Autodesk Inventor part; units mm, degrees
ref_plane "YZ Plane" through (0, 0, 0) normal (1, 0, 0) x (0, 1, 0)
ref_plane "XZ Plane" through (0, 0, 0) normal (0, 1, 0) x (-1, 0, 0)
ref_plane "XY Plane" through (0, 0, 0) normal (0, 0, 1) x (1, 0, 0)
sketch "Эскиз1" plane through (0, 0, 0) normal (0, 0, 1) x (1, 0, 0)
  line L0 (0, 0) -> (45, 0)
  line L1 (45, 0) -> (45, 20)
  line L2 (45, 20) -> (0, 20)
  line L3 (0, 20) -> (0, 0)
  dimension "d0" = 45
  dimension "d1" = 20
extrude "Выдавливание1" add sketch "Эскиз1" along normal blind 1.2
sketch "Эскиз2" plane through (0, 0, 1.2) normal (0, 0, 1) x (1, 0, 0)
  line L0 (0, 20) -> (0, 0)
  line L1 (0, 10) -> (1.5, 10)
  line L2 (1.5, 10) -> (9.5, 10)
  circle A0 centre (9.5, 10) radius 8
  line L3 (45, 20) -> (0, 20)
  line L4 (22.5, 20) -> (22.5, 0)
  line L5 (0, 0) -> (45, 0)
  circle A1 centre (35.5, 10) radius 8
  dimension "d5" = 16
  dimension "d4" = 1.5
extrude "Выдавливание2" add sketch "Эскиз2" along normal blind 13.8 contours A0 | A1
sketch "Эскиз3" plane through (0, 0, 1.2) normal (0, 0, 1) x (1, 0, 0)
  line L0 (45, 20) -> (0, 20)
  line L1 (22.5, 20) -> (22.5, 19.5)
  line L2 (27.5, 17.75) -> (17.5, 17.75) construction
  line L3 (25.75, 19.5) -> (19.25, 19.5)
  line L4 (19.25, 16) -> (25.75, 16)
  arc A0 (25.75, 16) -> (25.75, 19.5) centre (25.75, 17.75) ccw
  arc A1 (19.25, 19.5) -> (19.25, 16) centre (19.25, 17.75) ccw
  point P0 (0, 0)
  point P1 (22.5, 17.75)
  dimension "d8" = 0.5
  dimension "d9" = 10
  dimension "d10" = 3.5
extrude "Выдавливание3" add sketch "Эскиз3" along normal blind 3.3
sketch "Эскиз8" plane through (0, 0, 0) normal (0, 0, -1) x (-1, 0, 0)
  line L0 (-45, 0) -> (-45, 20)
  line L1 (-45, 20) -> (-44, 20)
  line L2 (-45, 20) -> (0, 20)
  line L3 (-44, 20) -> (-44, 19)
  circle A0 centre (-44, 19) radius 0.5
  line L4 (-45, 10) -> (0, 10)
  line L5 (0, 20) -> (0, 0)
  line L6 (-22.5, 20) -> (-22.5, 0)
  line L7 (0, 0) -> (-45, 0)
  circle A1 centre (-44, 1) radius 0.5
  circle A2 centre (-1, 19) radius 0.5
  circle A3 centre (-1, 1) radius 0.5
  dimension "d41" = 1
  dimension "d42" = 1
  dimension "d43" = 1
extrude "Выдавливание8" cut sketch "Эскиз8" against normal through all contours A0 | A1 | A2 | A3
sketch "Эскиз4" plane through (0, 0, 0) normal (0, 0, -1) x (-1, 0, 0)
  line L0 (-27.5, 2.5) -> (-17.5, 2.5)
  line L1 (-17.5, 2.5) -> (-17.5, 0)
  line L2 (-17.5, 0) -> (-27.5, 0)
  line L3 (-27.5, 0) -> (-27.5, 2.5)
  line L4 (-27.5, 2.5) -> (-17.5, 0) construction
  line L5 (-17.5, 2.5) -> (-27.5, 0) construction
  line L6 (0, 0) -> (-45, 0)
  point P0 (-22.5, 1.25)
  point P1 (-22.5, 0)
  dimension "d13" = 10
  dimension "d14" = 2.5
extrude "Выдавливание4" add sketch "Эскиз4" along normal blind 3.3
sketch "Эскиз5" plane through (0, 0, -3.3) normal (0, 0, -1) x (-1, 0, 0)
  line L0 (-26.5, 1.5) -> (-26, 1.5)
  line L1 (-26, 1.5) -> (-26, 1)
  line L2 (-26, 1) -> (-26.5, 1)
  line L3 (-26.5, 1) -> (-26.5, 1.5)
  line L4 (-26.5, 1.25) -> (-27.5, 1.25)
  line L5 (-27.5, 2.5) -> (-27.5, 0)
  line L6 (-24, 1.5) -> (-23.5, 1.5)
  line L7 (-23.5, 1.5) -> (-23.5, 1)
  line L8 (-23.5, 1) -> (-24, 1)
  line L9 (-24, 1) -> (-24, 1.5)
  line L10 (-21.5, 1.5) -> (-21, 1.5)
  line L11 (-21, 1.5) -> (-21, 1)
  line L12 (-21, 1) -> (-21.5, 1)
  line L13 (-21.5, 1) -> (-21.5, 1.5)
  line L14 (-19, 1.5) -> (-18.5, 1.5)
  line L15 (-18.5, 1.5) -> (-18.5, 1)
  line L16 (-18.5, 1) -> (-19, 1)
  line L17 (-19, 1) -> (-19, 1.5)
  point P0 (0, 0)
  point P1 (-24, 1.25)
  point P2 (-21.5, 1.25)
  point P3 (-19, 1.25)
  dimension "d17" = 0.5
  dimension "d18" = 0.5
  dimension "d19" = 1
  dimension "d22" = 2.5
extrude "Выдавливание5" add sketch "Эскиз5" along normal blind 2
sketch "Эскиз6" plane through (26, 1, -3.3) normal (0, -1, 0) x (1, 0, 0)
  line L0 (0.5, -2) -> (0, -2)
  line L1 (0, 0) -> (0, -2)
  line L2 (0.5, -2) -> (0, -2)
  line L3 (0, -2) -> (0, -1.5)
  line L4 (0, -1.5) -> (0.5, -1.5)
  line L5 (0.5, -1.5) -> (0.5, -2)
  line L6 (-2, -2) -> (-2.5, -2)
  line L7 (-2.5, -2) -> (-2.5, -1.5)
  line L8 (-2.5, -1.5) -> (-2, -1.5)
  line L9 (-2, -1.5) -> (-2, -2)
  line L10 (-4.5, -2) -> (-5, -2)
  line L11 (-5, -2) -> (-5, -1.5)
  line L12 (-5, -1.5) -> (-4.5, -1.5)
  line L13 (-4.5, -1.5) -> (-4.5, -2)
  line L14 (-7, -2) -> (-7.5, -2)
  line L15 (-7.5, -2) -> (-7.5, -1.5)
  line L16 (-7.5, -1.5) -> (-7, -1.5)
  line L17 (-7, -1.5) -> (-7, -2)
  point P0 (-26, 3.3)
  dimension "d31" = 2.5
extrude "Выдавливание6" add sketch "Эскиз6" along normal blind 7
sketch "Эскиз7" plane through (0, 0, 1.2) normal (0, 0, 1) x (1, 0, 0)
  line L0 (26.5, 1.5) -> (26, 1.5)
  line L1 (26.5, 1) -> (26.5, 1.5)
  line L2 (26, 1.5) -> (26, 1)
  line L3 (26, 1) -> (26.5, 1)
  line L4 (21, 1) -> (21.5, 1)
  line L5 (21.5, 1) -> (21.5, 1.5)
  line L6 (21.5, 1.5) -> (21, 1.5)
  line L7 (21, 1.5) -> (21, 1)
  line L8 (26.5, 1.5) -> (26, 1.5)
  line L9 (26, 1.5) -> (26, 1)
  line L10 (26, 1) -> (26.5, 1)
  line L11 (26.5, 1) -> (26.5, 1.5)
  line L12 (23.5, 1) -> (24, 1)
  line L13 (24, 1) -> (24, 1.5)
  line L14 (24, 1.5) -> (23.5, 1.5)
  line L15 (23.5, 1.5) -> (23.5, 1)
  line L16 (18.5, 1) -> (19, 1)
  line L17 (19, 1) -> (19, 1.5)
  line L18 (19, 1.5) -> (18.5, 1.5)
  line L19 (18.5, 1.5) -> (18.5, 1)
  line L20 (17.5, 0) -> (17.5, 2.5)
  line L21 (17.5, 2.5) -> (27.5, 2.5)
  line L22 (27.5, 2.5) -> (27.5, 0)
  line L23 (27.5, 0) -> (17.5, 0)
  point P0 (0, 0)
extrude "Выдавливание7" add sketch "Эскиз7" along normal blind 1.8 contours L1 L3 L2 L0 | L7 L6 L5 L4 | L15 L14 L13 L12 | L19 L18 L17 L16
fillet "Сопряжение1" radius 0.5 16 edges at (21.25, 1.5, 1.2) (21.25, 1, 1.2) (21.5, 1.25, 1.2) (21, 1.25, 1.2) (18.75, 1, 1.2) (18.5, 1.25, 1.2) (19, 1.25, 1.2) (18.75, 1.5, 1.2) (23.75, 1, 1.2) (24, 1.25, 1.2) (23.5, 1.25, 1.2) (23.75, 1.5, 1.2) (26.25, 1.5, 1.2) (26, 1.25, 1.2) (26.25, 1, 1.2) (26.5, 1.25, 1.2)
properties part number "Ultrasonic HC-SRO4"
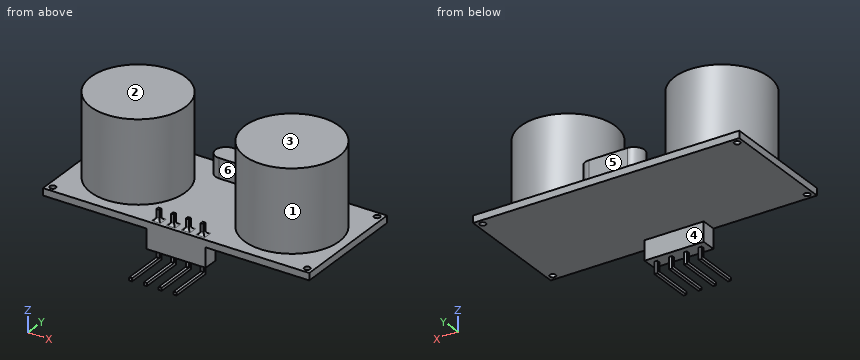
Geometry: final body of the model. Coordinates: model frame, mm. Face numbers are marked on the shaded views. A direction names the side the tool comes from. Give positions to 0.01 mm unless a question says otherwise; leave off trailing zeros. Order: outer loops, then holes, each group sorted by start corner. A loop starts at its lowest first (then second) coordinate and runs counter-clockwise, first axis right, second up. Notation, with made-up numbers: (1, -14) -> (33, -14) arc R18 cw to (33, -7) -> close; hole circle Ø9 at (26, -19.75). An arc over 180 degrees is marked (long way). Write each question's results on one line, items separated by ' | '. Start each with the question number.
1) Section D-D (y = 10.5). Return loops of the section in (x, z).
2) First-contact query: pin 1 (8 mm diameter, centred on x = 12.5, z = 8, fed in from +Y); pin 2 (3.5 mm diameter, centred on x = 24, z = 2.5, fed in from -Y); pin 3 (2 mm diameter, centred on y = -0.5, z = -4, fed in from +X); pin 4 (1 mm diameter, centred on y = 1, z = 4.5, fed in from -X). Flat tips, straight axial feed; report the tip coordinate or a pass-through.
3) Line query: line 1 (Y direction, x = 44, z = 0.95); line 2 (Z direction, x = 31.5, y = 10.5); line 3 (Z direction, x = 26.5, y = 5). Output: solid intervals per line, ascending. Write a range as from..to.
4) Draft query along X for the marked faces 1 and 2. Return one class per face: pulls with the +X half, pulls with the -X half, needs draft (parallel to the pull), parting line crosses it, or undercut.
5) Section B-B (z = 0.75). Return loops of the section in (x, y), then the cut area to 3 significant figures.
6) Set-up query: the marked faces 3, 4, 5 and 6. Return all of +Z, -Z, +X, -X, +Y, -Y with unobstructed straight access to the full face (end or side cutting, diameter ignored); none if empty.
7) Section A-A (x = 44). Return loops of the section in (y, z), then the cut area to 3 significant figures.
8) Section C-C (x = 35.5). Return loops of the section in (y, z), then the cut area to 3 significant figures.
Calculated:
1) outline: (0, 0) -> (45, 0) -> (45, 1.2) -> (43.48, 1.2) -> (43.48, 15) -> (27.52, 15) -> (27.52, 1.2) -> (17.48, 1.2) -> (17.48, 15) -> (1.52, 15) -> (1.52, 1.2) -> (0, 1.2) -> close
2) pin 1: y = 18 | pin 2: y = 0 | pin 3: x = 27.5 | pin 4: through
3) line 1: 0..0.5, 1.5..18.5, 19.5..20 | line 2: 0..15 | line 3: 0..1.2
4) face 1: undercut | face 2: needs draft
5) outline: (0, 0) -> (45, 0) -> (45, 20) -> (0, 20) -> close; hole circle Ø1 at (1, 1); hole circle Ø1 at (1, 19); hole circle Ø1 at (44, 1); hole circle Ø1 at (44, 19) | area: 897 mm2
6) face 3: +Z, +X, -X, +Y, -Y | face 4: -Z, +X, -X, +Y | face 5: +Z, +X, -X, +Y | face 6: +Z
7) outline: (0, 0) -> (0.5, 0) -> (0.5, 1.2) -> (0, 1.2) -> close; (1.5, 0) -> (18.5, 0) -> (18.5, 1.2) -> (1.5, 1.2) -> close; (19.5, 0) -> (20, 0) -> (20, 1.2) -> (19.5, 1.2) -> close | area: 21.6 mm2
8) outline: (0, 0) -> (20, 0) -> (20, 1.2) -> (18, 1.2) -> (18, 15) -> (2, 15) -> (2, 1.2) -> (0, 1.2) -> close | area: 245 mm2
